Can you work these out from the model? Positions are in its coordinate system, mm. A direction names the side the tool comes from. Round coordinates to 2 decimals unless told otherwise and drop trailing zeros. Loops run counter-clockwise (first coordinate to the right, second up) from the corner with the lowest first, then second, coordinate; pieces in that order, holes last.
```python
from build123d import *

# Parameters (mm, degrees)
SKETCH1_W           = 8
SKETCH1_H           = 7
BOSS_EXTRUDE3_DEPTH = 8
CUT_EXTRUDE1_DEPTH  = 8
CUT_EXTRUDE2_DEPTH  = 1
CUT_EXTRUDE4_DEPTH  = 2
CUT_EXTRUDE5_DEPTH  = 9
SKETCH7_OUTSIDE_W   = 12.66
SKETCH7_OUTSIDE_H   = 12.66
SKETCH7_OUTSIDE_W_2 = 4
SKETCH7_OUTSIDE_H_2 = 3
CUT_EXTRUDE6_DEPTH  = 2
SKETCH8_W           = 1
SKETCH8_H           = 1
CUT_EXTRUDE7_DEPTH  = 3
CUT_EXTRUDE8_DEPTH  = 5
SKETCH11_W          = 4
SKETCH11_H          = 2.236067977
CUT_EXTRUDE9_DEPTH  = 5
CUT_EXTRUDE10_DEPTH = 5
SKETCH13_W          = 2
SKETCH13_H          = 2
CUT_EXTRUDE12_DEPTH = 3


with BuildPart() as part:
    # Sketch1 → Boss-Extrude3 (new body)
    with BuildSketch(Plane.XY):
        Rectangle(SKETCH1_W, SKETCH1_H)
    extrude(amount=BOSS_EXTRUDE3_DEPTH)

    # Sketch3 → Cut-Extrude1 (cut, through all)
    with BuildSketch(Plane(origin=(0, 3.5, 0), x_dir=(1, 0, 0), z_dir=(0, 1, 0))):
        Polygon((4, -8), (4, -2), (3, -2), (3, -5), (1, -7), (-1, -7), (-1, -8), align=None)
    extrude(amount=-CUT_EXTRUDE1_DEPTH, mode=Mode.SUBTRACT)

    # Sketch4 → Cut-Extrude2 (cut)
    with BuildSketch(Plane.XZ.offset(3.5)):
        Polygon((1, 7), (3, 5), (3, 3), (0, 3), (0, 7), align=None)
    extrude(amount=-CUT_EXTRUDE2_DEPTH, mode=Mode.SUBTRACT)

    # Sketch5 → Cut-Extrude4 (cut)
    with BuildSketch(Plane(origin=(0, 0, 0), x_dir=(-1, 0, 0), z_dir=(0, 0, -1))):
        Polygon((-2, -0.5), (-2, 1.5), (-2, 3.5), (-4, 3.5), (-4, 1.5), (-4, -2.5), align=None)
    extrude(amount=-CUT_EXTRUDE4_DEPTH, mode=Mode.SUBTRACT)

    # Sketch6 → Cut-Extrude5 (cut, through all)
    with BuildSketch(Plane.ZY.offset(4)):
        Polygon((8, -1.5), (7, -1.5), (5, 1.5), (5, 3.5), (8, 3.5), align=None)
    extrude(amount=-CUT_EXTRUDE5_DEPTH, mode=Mode.SUBTRACT)

    # Sketch7 outside → Cut-Extrude6 (cut)
    with BuildSketch(Plane(origin=(0, 3.5, 0), x_dir=(1, 0, 0), z_dir=(0, 1, 0))):
        with Locations((0, -4)):
            Rectangle(SKETCH7_OUTSIDE_W, SKETCH7_OUTSIDE_H)
        with Locations((-1, -2.5)):
            Rectangle(SKETCH7_OUTSIDE_W_2, SKETCH7_OUTSIDE_H_2, mode=Mode.SUBTRACT)
    extrude(amount=-CUT_EXTRUDE6_DEPTH, mode=Mode.SUBTRACT)

    # Sketch8 → Cut-Extrude7 (cut)
    with BuildSketch(Plane(origin=(0, 1.5, 0), x_dir=(1, 0, 0), z_dir=(0, 1, 0))):
        with Locations((-1.5, -6.5)):
            Rectangle(SKETCH8_W, SKETCH8_H)
    extrude(amount=-CUT_EXTRUDE7_DEPTH, mode=Mode.SUBTRACT)

    # Sketch9 → Cut-Extrude8 (cut)
    with BuildSketch(Plane(origin=(0, 3.5, 0), x_dir=(1, 0, 0), z_dir=(0, 1, 0))):
        Polygon((-1, -6), (-1, -4), (3, -4), (3, -7), (-1, -7), align=None)
    extrude(amount=-CUT_EXTRUDE8_DEPTH, mode=Mode.SUBTRACT)

    # Sketch11 → Cut-Extrude9 (cut)
    with BuildSketch(Plane(origin=(0, 1.9, 3.8), x_dir=(1, 0, 0), z_dir=(0, 0.447213595, 0.894427191))):
        with Locations((-1, 0.670820394)):
            Rectangle(SKETCH11_W, SKETCH11_H)
    extrude(amount=CUT_EXTRUDE9_DEPTH, mode=Mode.SUBTRACT)

    # Sketch12 → Cut-Extrude10 (cut)
    with BuildSketch(Plane(origin=(0, 3.5, 0), x_dir=(1, 0, 0), z_dir=(0, 1, 0))):
        Polygon((1, -2), (-1, -4), (1, -4), align=None)
    extrude(amount=-CUT_EXTRUDE10_DEPTH, mode=Mode.SUBTRACT)

    # Sketch13 → Cut-Extrude12 (cut)
    with BuildSketch(Plane(origin=(0, 1.5, 0), x_dir=(1, 0, 0), z_dir=(0, 1, 0))):
        with Locations((2, -3)):
            Rectangle(SKETCH13_W, SKETCH13_H)
    extrude(amount=-CUT_EXTRUDE12_DEPTH, mode=Mode.SUBTRACT)


solid = part.part
```
(1) Suppose I cut it at B-B (x = -2.25). Write out the boundary of the cut face in (y, z).
(2) Which directions (+Z, -Z, +X, -X, +Y, -Y) give clear straight access to the entire face, cutting with the end or side of a thin tool? Please do faces 1 (the flat face through (0, -3, 5)), 2 (the flat face through (1.5, 0, 2)), 3 (the flat face through (-3, 3, 2)), 4 (the flat face through (3.5, -2.7, 2)).
(3) If I drill on line 1 (X direction, y = -1.75, z = 3.75); line 2 (Y direction, x = 1, z = 0.5); line 3 (Y direction, x = 1.5, z = 4), over which ranges is the centre line in solid material (lowest first)?
(4) Suppose I cut it at A-A (z = 2.25). Write out the boundary of the cut face in (x, y), then the cut area to 4 significant figures.
(5) For pin 1 (0.5 mm diameter, centred on y = -2, z = 7.5, fed in from +X); pin 2 (1.6 mm diameter, centred on x = 0.5, y = -3, fed in from +Z); pin 3 (0.5 mm diameter, centred on x = 1.5, y = -3, fed in from +Z), each with a flat end and sliding along its axis, tell me the tip position at first contact or that it passes through.
(6) Suppose I cut it at D-D (z = 5.5). Write out the boundary of the cut face in (x, y), then the cut area to 4 significant figures.
(7) Suppose I cut it at C-C (y = -1.75). Write out the boundary of the cut face in (x, z), then the cut area to 3 significant figures.
Check result:
1. outline: (-3.5, 0) - (1.5, 0) - (1.5, 1) - (3.5, 1) - (3.5, 3) - (1.5, 4) - (1.5, 5) - (-1.5, 7) - (-1.5, 8) - (-3.5, 8) - close
2. face 1: +Z, +X, -Y
2. face 2: +Z, +X, +Y
2. face 3: +Z, -Z, -X, +Y
2. face 4: +Z, +X, +Y, -Y
3. line 1: x = -4 to 3
3. line 2: y = -3.5 to 1.5
3. line 3: y = -2.5 to -1.5
4. outline: (-4, -3.5) - (3, -3.5) - (3, -1.5) - (0.75, -1.5) - (0.75, 3.5) - (-3, 3.5) - (-3, 1.5) - (-4, 1.5) - close
4. area: 35.75 mm2
5. pin 1: stops at x = -1
5. pin 2: stops at z = 7
5. pin 3: stops at z = 3
6. outline: (-4, -3.5) - (0, -3.5) - (0, -2.5) - (2.5, -2.5) - (2.5, -1.5) - (-1, -1.5) - (-1, 0.75) - (-4, 0.75) - close
6. area: 17.25 mm2
7. outline: (-4, 0) - (3.25, 0) - (3.25, 2) - (3, 2) - (3, 5) - (1, 7) - (-1, 7) - (-1, 8) - (-4, 8) - close
7. area: 50.5 mm2
